Geometry: see drawing. Coordinates: mm, zero at the bounding-box minimum. A direction names the side the tool comes from. Coordinates: 2 decimals unless noted, no trailing zeros. Order: outer loops, then holes, each group sorted by start corner. A loop starts at its lowest first (then second) coordinate and runs counter-clockwise, first axis right, second up. Notation, with made-up numbers: (51, -39.5) -> (109, -39.5) arc R21 cw to (109, -20.5) -> close; hole circle Ø10 at (-17.75, 54.5). An arc over 180 degrees is marked (long way). Write each question's results on one line, items separated by ' | '. Start each with the question number.
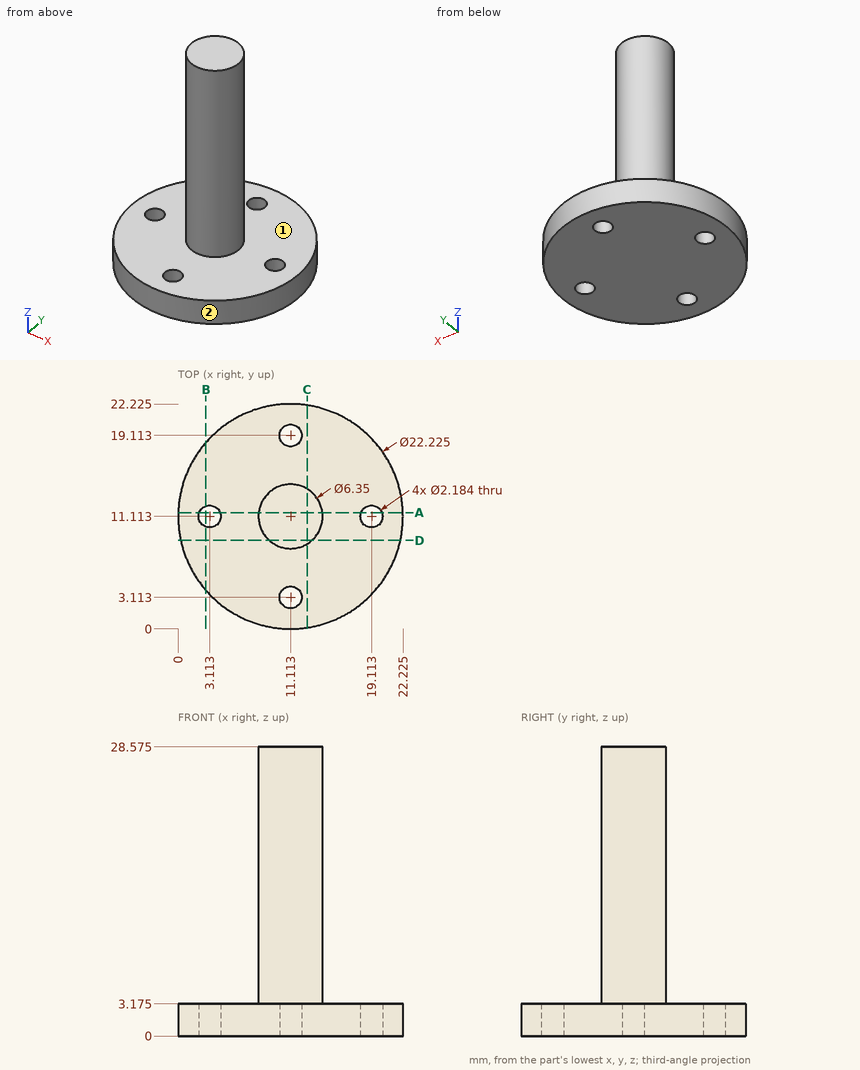
(1) Section A-A on y = 11.5. Return the cut outline in (x, z) (1 decimal).
(2) Section B-B on x = 2.75. Return the cut outline in (y, z) (1 decimal).
(3) Section D-D on y = 8.75. Return the cut outline in (x, z) (1 decimal).
(4) Reachability of the marked faces 1 and 2 from +Z, -Z, +X, -X, +Y, -Y: full face, straight path, thin tool, end or side. Return the list, or none.
(5) Section C-C on x = 12.75. Return the cut outline in (y, z) (1 decimal).
(6) First-contact query: P1, Ø5, axis at y = 15.5, z = 9.5, coming from the -X side; P2, Ø4, axis at y = 14.5, z = 17.5, coming from the -X side; P3, Ø1, axis at y = 8.5, z = 22, coming from the -X side; P4, Ø1.3, axis at x = 19.11, y = 11.11, coming from the +Z side. Flat tips, straight axial feed; report the tip coordinate or a pass-through.
(7) Line query: L1, parallel to Z at x = 6.5, y = 19.25 (1 decimal); L2, parallel to Y at x = 10, z = 12.75 (1 decimal); L3, parallel to Y at x = 8.25, z = 27.5 (1 decimal). Output: solid intervals per line, ascending.
Results list:
1) outline: (0, 0) -> (2.1, 0) -> (2.1, 3.2) -> (0, 3.2) -> close; (4.1, 0) -> (18.1, 0) -> (18.1, 3.2) -> (14.3, 3.2) -> (14.3, 28.6) -> (8, 28.6) -> (8, 3.2) -> (4.1, 3.2) -> close; (20.1, 0) -> (22.2, 0) -> (22.2, 3.2) -> (20.1, 3.2) -> close
2) outline: (3.8, 0) -> (10.1, 0) -> (10.1, 3.2) -> (3.8, 3.2) -> close; (12.1, 0) -> (18.4, 0) -> (18.4, 3.2) -> (12.1, 3.2) -> close
3) outline: (0.3, 0) -> (22, 0) -> (22, 3.2) -> (13.2, 3.2) -> (13.2, 28.6) -> (9, 28.6) -> (9, 3.2) -> (0.3, 3.2) -> close
4) face 1: +Z | face 2: +Z, -Z
5) outline: (0.1, 0) -> (22.1, 0) -> (22.1, 3.2) -> (13.8, 3.2) -> (13.8, 28.6) -> (8.4, 28.6) -> (8.4, 3.2) -> (0.1, 3.2) -> close
6) P1: stops at x = 8.56 | P2: stops at x = 8.26 | P3: stops at x = 8.74 | P4: passes through
7) L1: z = 0 to 3.2 | L2: y = 8.1 to 14.1 | L3: y = 9.7 to 12.5
